Autodesk Inventor part; units mm, degrees
ref_plane "YZ Plane" through (0, 0, 0) normal (1, 0, 0) x (0, 1, 0)
ref_plane "XZ Plane" through (0, 0, 0) normal (0, 1, 0) x (-1, 0, 0)
ref_plane "XY Plane" through (0, 0, 0) normal (0, 0, 1) x (1, 0, 0)
sketch "スケッチ2" plane through (0, 0, 0) normal (0, 0, 1) x (1, 0, 0)
  line L0 (-31.5, 15) -> (31.5, 15)
  line L1 (31.5, 15) -> (31.5, -15)
  line L2 (31.5, -15) -> (-31.5, -15)
  line L3 (-31.5, -15) -> (-31.5, 15)
  line L4 (0, 24.6) -> (0, -21.6) construction
  line L5 (-44.1, 0) -> (44.1, 0) construction
  line L6 (-31.5, 15) -> (31.5, 15)
  line L7 (31.5, 15) -> (31.5, 18)
  line L8 (31.5, 18) -> (-31.5, 18)
  line L9 (-31.5, 18) -> (-31.5, 15)
  point P0 (0, 0)
  point P1 (31.5, 15)
  dimension "d1" = 63
  dimension "d2" = 30
  dimension "d3" = 15
  dimension "d4" = 31.5
  dimension "d26" = 3
extrude "押し出し1" add sketch "スケッチ2" along normal blind 3
sketch "スケッチ3" plane through (0, 0, 3) normal (0, 0, 1) x (1, 0, 0)
  line L0 (-31.5, -15) -> (31.5, -15) construction
  line L1 (-44.1, 0) -> (44.1, 0) construction
  line L2 (31.5, -15) -> (31.5, 18)
  line L3 (31.5, 18) -> (-31.5, 18)
  line L4 (-31.5, 18) -> (-31.5, -15)
  point P0 (0, 0)
  point P1 (-16.5, 0)
  point P2 (16.5, 0)
hole "穴1" at (-16.5, 0, 3) at (16.5, 0, 3) direction (0, 0, -1) diameter 6.6 end through all
fillet "フィレット1" radius 2 4 edges at (31.5, -15, 1.5) (-31.5, -15, 1.5) (-31.5, 18, 1.5) (31.5, 18, 1.5)
sketch "スケッチ4" plane through (0, 0, 3) normal (0, 0, 1) x (1, 0, 0)
  line L0 (-29.5, -15) -> (29.5, -15)
  arc A0 (-31.5, -13) -> (-29.5, -15) centre (-29.5, -13) ccw
  line L1 (-29.5, -15) -> (29.5, -15)
  arc A1 (29.5, -15) -> (31.5, -13) centre (29.5, -13) ccw
  circle A2 centre (-16.5, 0) radius 3.3
  circle A3 centre (16.5, 0) radius 3.3
  line L2 (1.5, -11) -> (-1.5, -11)
  line L3 (-1.5, -11) -> (-1.5, 11)
  line L4 (-1.5, 11) -> (1.5, 11)
  line L5 (1.5, 11) -> (1.5, -11)
  line L6 (1.5, -11) -> (-1.5, 11) construction
  line L7 (-1.5, -11) -> (1.5, 11) construction
  line L8 (31.5, -13) -> (31.5, 16)
  line L9 (29.5, 18) -> (-29.5, 18)
  line L10 (-31.5, 16) -> (-31.5, -13)
  arc A4 (31.5, 16) -> (29.5, 18) centre (29.5, 16) ccw
  arc A5 (-29.5, 18) -> (-31.5, 16) centre (-29.5, 16) ccw
  point P0 (0, 0)
  dimension "d22" = 3
  dimension "d24" = 4
extrude "押し出し2" add sketch "スケッチ4" along normal blind 3 contours L2 L3 L4 L5
fillet "フィレット2" radius 1 2 edges at (-1.5, 0, 6) (1.5, 0, 6)
fillet "フィレット2" radius 0.5 4 edges at (0, 11, 3) (0, -11, 3) (0, 11, 6) (0, -11, 6)
equation "\"d3\" = 0.5 * d2"
equation "\"d4\" = 0.5 * d1"
equation "\"d24\" = d23"
properties part number "rocker_frame_mount_02"
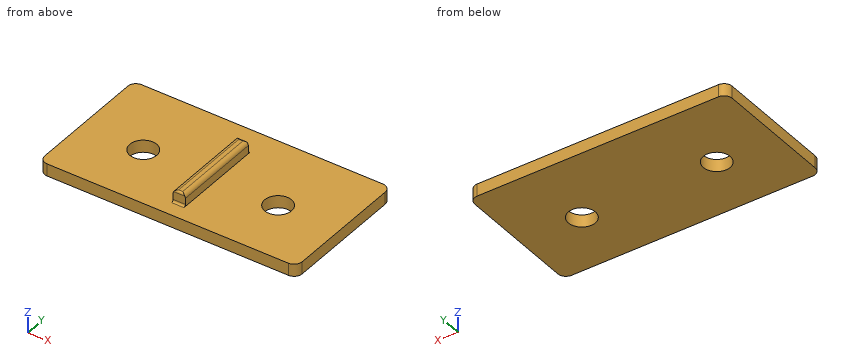
The listing builds one solid part. Answer for the finished solid, in the listing's coordinates (mm). Give positions to 0.01 mm unless a question says otherwise; leave off trailing zeros. Order: outer loops, then holes, each group sorted by start corner. A loop starts at its lowest first (then second) coordinate and runs counter-clockwise, first axis right, second up. Notation, with made-up numbers: (26, -16.5) -> (57, -16.5) arc R16 ccw to (57, -0.5) -> close; hole circle Ø8 at (70, 19). An arc over 180 degrees is marked (long way). Answer as CSV lines item,"result". Start each with the question number.
Q1. A cutting plane is placed at A-A (y = 0). Determine the outline of the cut face in (x, z), then the cut area to 3 significant figures.
Q2. Find the intervals of material crossed by L1, parallel to X at y = 0, z = 1.5; L2, parallel to Y at x = 16.5, z = 1.45; L3, parallel to Z at x = 4, y = -7.5, in increasing order.
Q3. A cutting plane is placed at B-B (x = -16.5). Determine the outline of the cut face in (y, z).
Q4. Given pin 1 (1.6 mm diameter, centred on y = 5, z = 4.5, fed in from -X); pin 2 (3 mm diameter, centred on x = -20.5, y = -8.5, fed in from +Z); pin 3 (1.6 mm diameter, centred on x = 0, z = 4.5, fed in from +Y); pin 4 (1 mm diameter, centred on x = 19, z = 4, fed in from -Y), each flat-ended and moving along its own axis, determine where each tip first touches the part or whether it passes through.
Q5. A cutting plane is placed at C-C (y = 8.5). Determine the outline of the cut face in (x, z), then the cut area to 3 significant figures.
Q6. A cutting plane is placed at D-D (x = 3). Determine the outline of the cut face in (y, z).
Results found:
1,outline,"(-31.5, 0) -> (-19.8, 0) -> (-19.8, 3) -> (-31.5, 3) -> close; (-13.2, 0) -> (13.2, 0) -> (13.2, 3) -> (1.5, 3) -> (1.5, 5) arc R1 ccw to (0.5, 6) -> (-0.5, 6) arc R1 ccw to (-1.5, 5) -> (-1.5, 3) -> (-13.2, 3) -> close; (19.8, 0) -> (31.5, 0) -> (31.5, 3) -> (19.8, 3) -> close"
1,area,"158 mm2"
2,L1,"-31.5 to -19.8, -13.2 to 13.2, 19.8 to 31.5"
2,L2,"-15 to -3.3, 3.3 to 18"
2,L3,"0 to 3"
3,outline,"(-15, 0) -> (-3.3, 0) -> (-3.3, 3) -> (-15, 3) -> close; (3.3, 0) -> (18, 0) -> (18, 3) -> (3.3, 3) -> close"
4,pin 1,"x = -1.5"
4,pin 2,"z = 3"
4,pin 3,"y = 11"
4,pin 4,"through"
5,outline,"(-31.5, 0) -> (31.5, 0) -> (31.5, 3) -> (1.5, 3) -> (1.5, 5) arc R1 ccw to (0.5, 6) -> (-0.5, 6) arc R1 ccw to (-1.5, 5) -> (-1.5, 3) -> (-31.5, 3) -> close"
5,area,"198 mm2"
6,outline,"(-15, 0) -> (18, 0) -> (18, 3) -> (-15, 3) -> close"
